Autodesk Inventor part; units mm, degrees
ref_plane "YZ Plane" through (0, 0, 0) normal (1, 0, 0) x (0, 1, 0)
ref_plane "XZ Plane" through (0, 0, 0) normal (0, 1, 0) x (-1, 0, 0)
ref_plane "XY Plane" through (0, 0, 0) normal (0, 0, 1) x (1, 0, 0)
sketch "スケッチ2" plane through (0, 0, 0) normal (0, 0, 1) x (1, 0, 0)
  line L0 (0, 0) -> (26, 0)
  line L1 (26, 0) -> (26, 33)
  line L2 (26, 33) -> (0, 33)
  line L3 (0, 33) -> (0, 0)
  line L4 (0, 0) -> (26, 0)
  line L5 (26, 0) -> (26, 24)
  line L6 (26, 24) -> (0, 24) construction
  line L7 (0, 24) -> (0, 0)
  circle A0 centre (13, 24) radius 13
  circle A1 centre (13, 24) radius 6.25
  line L8 (26, 0) -> (0, 0)
  line L9 (17.9352, 27.452) -> (40.6962, -11.9711)
  line L10 (40.6962, -11.9711) -> (18.1795, -24.9711)
  line L11 (18.1795, -24.9711) -> (-4.3205, 14)
  circle A2 centre (21.5096, -20.7391) radius 0.8
  circle A3 centre (35.366, -12.7391) radius 0.8
  line L12 (-4.3205, 14) -> (18.1962, 27)
  point P0 (22.3808, 33)
  point P1 (3.6192, 33)
  point P2 (26, 13.4833)
  point P3 (3.7624, 0)
  point P4 (23.9624, 17.0125)
  point P5 (1.7417, 17.5)
  point P6 (0, 16.4944)
  point P7 (0, 6.5167)
  point P8 (7.5873, 20.875)
  point P9 (19.0712, 25.4845)
  dimension "d0" = 26
  dimension "d1" = 33
  dimension "d2" = 24
  dimension "d3" = 12.5
  dimension "d14" = 26
  dimension "d17" = 1.6
  dimension "d18" = 1.6
  dimension "d19" = 2
  dimension "d20" = 2
  dimension "d21" = 5
  dimension "d22" = 5
  dimension "d23" = 20
  dimension "d25" = 45
  dimension "d26" = 30
extrude "押し出し1" add sketch "スケッチ2" along normal blind 1.5 contours L3 L11 L0 | L11 L3 L12 A0 L9 L1 L0 | L0 L1 L9 L10 L11 | L3 A0 L12 | L9 A0 L1 | A0 L2 L9 A1 L12 | L12 A1 L9 A0
sketch "スケッチ3" plane through (0, 0, 0) normal (0, 0, -1) x (-1, 0, 0)
  circle A0 centre (-2.5, 24) radius 0.85
  circle A1 centre (-23.5, 24) radius 0.85
  circle A2 centre (-23.5, 3) radius 0.85
  circle A3 centre (-2.5, 3) radius 0.85
  circle A4 centre (-30.366, -4.0788) radius 0.8
  circle A5 centre (-16.5096, -12.0788) radius 0.8
  circle A6 centre (-13, 24) radius 6.25
  line L0 (-2.5, 24) -> (-23.5, 24)
  line L1 (-23.5, 24) -> (-23.5, 3)
  line L2 (-23.5, 3) -> (-2.5, 3)
  line L3 (-2.5, 3) -> (-2.5, 24)
  circle A7 centre (-13, 24) radius 10.25
  line L4 (-5.5, 24) -> (-20.5, 24)
  line L5 (-20.5, 24) -> (-20.5, 3)
  line L6 (-20.5, 3) -> (-5.5, 3)
  line L7 (-5.5, 3) -> (-5.5, 24)
  line L8 (-3.7624, 0) -> (-18.1795, -24.9711)
  line L9 (0, 24) -> (0, 0)
  arc A8 (0, 24) -> (-3.6192, 33) centre (-13, 24) ccw
  line L10 (-22.3808, 33) -> (-3.6192, 33)
  arc A9 (-22.3808, 33) -> (-26, 24) centre (-13, 24) ccw
  line L11 (-26, 13.4833) -> (-26, 24)
  line L12 (-40.6962, -11.9711) -> (-26, 13.4833)
  line L13 (-18.1795, -24.9711) -> (-40.6962, -11.9711)
  line L14 (-3.7624, 0) -> (-18.1795, -24.9711)
  line L15 (0, 0) -> (-3.7624, 0)
  circle A10 centre (-13, 24) radius 6.25
  circle A11 centre (-21.5096, -20.7391) radius 0.8
  circle A12 centre (-35.366, -12.7391) radius 0.8
  line L16 (-21.5096, -20.7391) -> (-16.5096, -12.0788)
  line L17 (-16.5096, -12.0788) -> (-30.366, -4.0788)
  line L18 (-30.366, -4.0788) -> (-35.366, -12.7391)
  line L19 (-35.366, -12.7391) -> (-21.5096, -20.7391)
  line L20 (-22.2417, -18.007) -> (-19.2417, -12.8109)
  line L21 (-19.2417, -12.8109) -> (-29.634, -6.8109)
  line L22 (-29.634, -6.8109) -> (-32.634, -12.007)
  line L23 (-32.634, -12.007) -> (-22.2417, -18.007)
  line L24 (-13.2817, -10.4784) -> (-24.5317, -3.9832)
  line L25 (-24.5317, -3.9832) -> (-16.75, 9.4952)
  line L26 (-16.75, 9.4952) -> (-5.5, 3)
  line L27 (-5.5, 3) -> (-13.2817, -10.4784)
  line L28 (-24.5317, -3.9832) -> (-28.866, -1.4808)
  line L29 (-28.866, -1.4808) -> (-28.0111, 0)
  line L30 (-28.0111, 0) -> (-22.2321, 0)
  line L31 (-22.2321, 0) -> (-7.2321, 0)
  point P0 (-5.5, 17.0134)
  point P1 (-20.5, 17.0134)
  dimension "d27" = 4
  dimension "d28" = 3
  dimension "d29" = 3
  dimension "d31" = 2
  dimension "d32" = 2
  dimension "d33" = 2
  dimension "d34" = 2
  dimension "d35" = 3
  dimension "d36" = 3
extrude "押し出し2" cut sketch "スケッチ3" against normal through all contours A0 L3 L0 A7 | A7 L0 A0 | A0 A7 L0 L3 | L0 A7 A0 | L3 L2 A3 | A3 L2 L3 | L7 L26 L25 L5 A7 | A7 L0 L1 A1 | A1 L0 A7 | L2 L25 L26 | A1 A7 L0 | L1 L0 A7 A1 | L27 L24 L25 L31 | L1 L2 A2 | A2 L2 L1 | L25 L28 L29 L30 | A4 L17 L18 | L18 L17 A4 | L17 L16 A5 | A5 L16 L17 | L23 L22 L21 L20
fillet "フィレット1" radius 3 19 edges at (20.5, 3, 0.75) (5.5, 3, 0.75) (20.5, 17.0134, 0.75) (5.5, 17.0134, 0.75) (7.2321, 0, 0.75) (13.2817, -10.4784, 0.75) (28.0111, 0, 0.75) (28.866, -1.4808, 0.75) (29.634, -6.8109, 0.75) (32.634, -12.007, 0.75) (22.2417, -18.007, 0.75) (19.2417, -12.8109, 0.75) (40.6962, -11.9711, 0.75) (18.1795, -24.9711, 0.75) (3.7624, 0, 0.75) (0, 0, 0.75) (26, 13.4833, 0.75) (22.3808, 33, 0.75) (3.6192, 33, 0.75)
equation "\"d20\" = d19"
properties part number "elbow" material "アルミニウム 6061"
Work out the finished part from the listing and answer in its coordinate system (mm). A direction names the side the tool comes from. Give positions to 0.01 mm unless a question says otherwise; leave off trailing zeros. Write each loop counter-clockwise with the first axis right and the second up, starting at its lowest first coordinate (ties: lowest second). Pieces come first, ordered by that corner, then holes. Notation, with made-up numbers: (-26, -30.5) - (26, -30.5) arc R23 ccw to (26, 1.5) - close; hole circle Ø8 at (81, 12). An arc over 180 degrees is marked (long way). Use one line per item in the form item = value.
1. A cutting plane is placed at C-C (z = 0.25). State how many separate pieces and enclosed holes the cut face has, and give its area (3 significant figures).
Filled in:
separate_pieces = 1
enclosed_holes = 12
area = 977 mm^2
2. Determine the mould class of faces 3 (the face through (26, 19, 1)), 4 (the face through (20.5, 9, 1)), 5 (the face through (25.314, 28.166, 0.74)) for opening direction Y: released by +Y, released by -Y, zero draft, split by the parting line, or undercut.
Filled in:
face_3 = zero draft
face_4 = undercut
face_5 = released by +Y
3. A cutting plane is placed at B-B (x = 13). Write down the section's boundary in (y, z), and give its area (3 significant figures).
Filled in:
outline = (-16, 0) - (-9.04, 0) - (-9.04, 1.5) - (-16, 1.5) - close; (0, 0) - (3, 0) - (3, 1.5) - (0, 1.5) - close; (13.75, 0) - (17.75, 0) - (17.75, 1.5) - (13.75, 1.5) - close; (30.25, 0) - (33, 0) - (33, 1.5) - (30.25, 1.5) - close
area = 25.1 mm^2
4. For faces 1 (the face through (10.738, -12.083, 0.74)), 2 (the face through (18.77, -7.31, 0.74)), determine the directions among +Z, -Z, +X, -X, +Y, -Y from which every point of the face is accessible in a straight line to the end or side of a thin tool.
Filled in:
face_1 = +Z, -Z, -X, -Y
face_2 = +Z, -Z
5. Consider L1, parallel to X at y = 24, z = 0.8; L2, parallel to X at y = 6.5, z = 0.4; L3, parallel to Y at x = 18.5, z = 0.7. Determine where each line is inside the solid, lowest interval first.
Filled in:
L1 = 0 to 1.65, 3.35 to 6.75, 19.25 to 22.65, 24.35 to 26
L2 = 0 to 5.5, 20.5 to 30.03
L3 = -23.77 to -7.47, 0 to 3.17, 14.37 to 21.03, 26.97 to 33
6. This flat-tipped pin is pushed along its axis until it touches: pin 1 Ø7.5 at (x, y) = (13, 24) entering from +Z. Where does it stop, or does it pass through?
Filled in:
pin_1 = through
7. A cutting plane is placed at A-A (y = 22.5). Write down the section's boundary in (x, z).
Filled in:
outline = (0, 0) - (6.93, 0) - (6.93, 1.5) - (0, 1.5) - close; (19.07, 0) - (26, 0) - (26, 1.5) - (19.07, 1.5) - close
